Can you work these out from the drawing? Everything is in mm from the part's minimum corner. Round coordinates to 2 decimals unless told otherwise and drop trailing zeros. Order: outer loops, then holes, each group sorted by start corner. A loop starts at its lowest first (then second) coordinate and runs counter-clockwise, first axis right, second up. Notation, with made-up numbers: (-15.5, 28.25) -> (-2.5, 28.25) arc R29 cw to (-2.5, 52.25) -> close; hole circle Ø1 at (39.5, 65.25). An arc over 180 degrees is marked (long way). One line per item, written item: value.
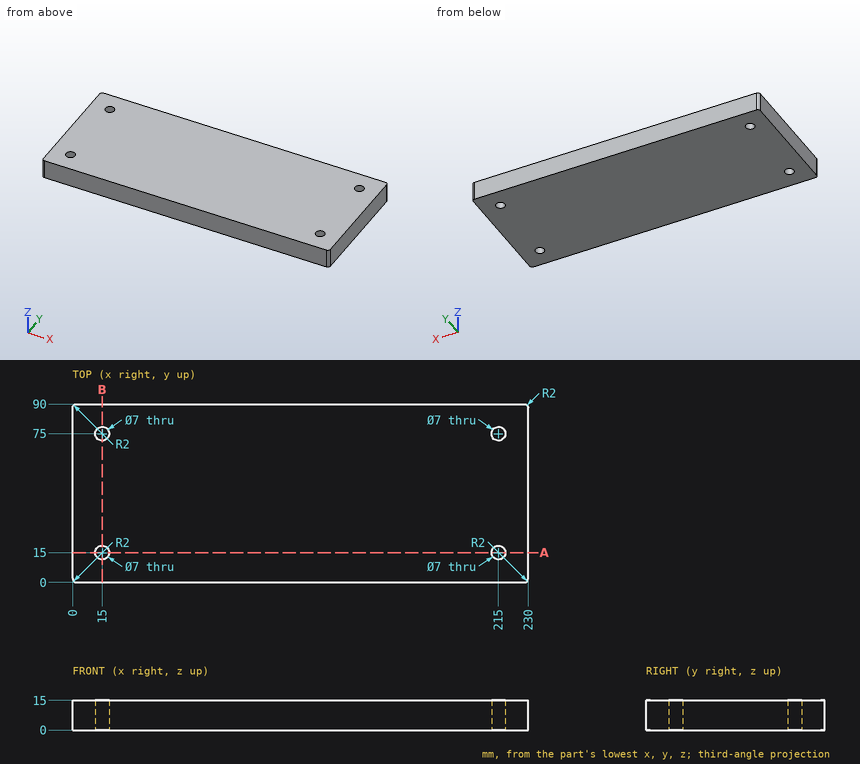
Q1. I want a section at A-A on y = 15. Write out the boundary of the cut face in (x, z), then the cut area to 3 significant figures.
Answers:
outline: (0, 0) -> (11.5, 0) -> (11.5, 15) -> (0, 15) -> close; (18.5, 0) -> (211.5, 0) -> (211.5, 15) -> (18.5, 15) -> close; (218.5, 0) -> (230, 0) -> (230, 15) -> (218.5, 15) -> close
area: 3,240 mm2
Q2. I want a section at B-B on x = 15. Write out the boundary of the cut face in (y, z), then the cut area to 3 significant figures.
Answers:
outline: (0, 0) -> (11.5, 0) -> (11.5, 15) -> (0, 15) -> close; (18.5, 0) -> (71.5, 0) -> (71.5, 15) -> (18.5, 15) -> close; (78.5, 0) -> (90, 0) -> (90, 15) -> (78.5, 15) -> close
area: 1,140 mm2
Q3. I need wall thicknesses on line 1 along Y through (x, z) = (15, 11); line 2 along X through (y, z) = (12, 7.75); line 3 along X through (y, z) = (17, 10). Which ranges of each line are inside material? Lowest first, please.
Answers:
line 1: 0 to 11.5, 18.5 to 71.5, 78.5 to 90
line 2: 0 to 13.2, 16.8 to 213.2, 216.8 to 230
line 3: 0 to 12.13, 17.87 to 212.13, 217.87 to 230
